The listing builds one solid part. Answer for the finished solid, in the listing's coordinates (mm). Round coordinates to 2 decimals unless told otherwise and drop trailing zeros. Loops run counter-clockwise (first coordinate to the right, second up) from the corner with the lowest first, then second, coordinate; pieces in that order, holes last. Notation, with made-up numbers: (30, -18.75) - (82, -18.75) arc R15 ccw to (82, -8.75) - close; hole circle Ø8 at (75, 89). An arc over 180 degrees is marked (long way). One line per item, written item: value.
```python
from build123d import *

# Parameters (mm, degrees)
SKETCH1_2_R         = 1.6383
SKETCH1_2_R_2       = 0.8382
BOSS_EXTRUDE2_DEPTH = 1.575


with BuildPart() as part:
    # Sketch1_2 → Boss-Extrude2 (new body)
    with BuildSketch(Plane(origin=(0, 0, 0), x_dir=(1, 0, 0), z_dir=(0, 1, 0))):
        with BuildLine():
            Line((-38.39500299, 29.999999735), (-42.73000299, 29.999999735))
            Line((-42.73000299, 29.999999735), (-43.011025994, 30.003097626))
            ThreePointArc((-43.011025994, 30.003097626), (-43.710996344, 30.299838092), (-44.000003042, 31.003036872))
            Line((-44.000003042, 31.003036872), (-44.000003042, 31.269999735))
            Line((-44.000003042, 31.269999735), (-44.000005679, 44.999999735))
            ThreePointArc((-44.000005679, 44.999999735), (-43.414218633, 46.414215608), (-42.000002924, 47.000003051))
            Line((-42.000002924, 47.000003051), (-30.435003, 47.000003051))
            Line((-30.435003, 47.000003051), (-30.435003, 22.255357341))
            Line((-30.435003, 22.255357341), (-11.909003, 22.255357341))
            Line((-11.909003, 22.255357341), (-11.909003, -8.5))
            Line((-11.909003, -8.5), (-23.409003, -8.5))
            Line((-23.409003, -8.5), (-23.409003, -31.499996949))
            Line((-23.409003, -31.499996949), (23.408997, -31.499996949))
            Line((23.408997, -31.499996949), (23.408997, -8.499997555))
            Line((23.408997, -8.499997555), (11.97084713, -8.499997555))
            Line((11.97084713, -8.499997555), (11.97084713, 22.255357341))
            Line((11.97084713, 22.255357341), (30.434997, 22.255357341))
            Line((30.434997, 22.255357341), (30.434997, 47.000003051))
            Line((30.434997, 47.000003051), (42.000008541, 47.000003051))
            ThreePointArc((42.000008541, 47.000003051), (43.414213215, 46.414220704), (43.999996956, 45.000016607))
            Line((43.999996956, 45.000016607), (43.999996956, 32.000003378))
            Line((43.999996956, 32.000003378), (43.999996956, 31.015615364))
            ThreePointArc((43.999996956, 31.015615364), (43.706534093, 30.307939396), (42.998386406, 30.015616661))
            Line((42.998386406, 30.015616661), (33.825607551, 30.030389905))
            ThreePointArc((33.825607551, 30.030389905), (33.117459864, 29.738067169), (32.823997, 29.030391202))
            Line((32.823997, 29.030391202), (32.823997, -30.453996949))
            ThreePointArc((32.823997, -30.453996949), (33.116890219, -31.16110373), (33.823997, -31.453996949))
            Line((33.823997, -31.453996949), (36.099999555, -31.453996949))
            Line((36.099999555, -31.453996949), (42.849728118, -31.453996949))
            ThreePointArc((42.849728118, -31.453996949), (43.556834899, -31.746890168), (43.849728118, -32.453996949))
            Line((43.849728118, -32.453996949), (43.849728118, -36.999996949))
            Line((43.849728118, -36.999996949), (43.849728118, -46.999996949))
            Line((43.849728118, -46.999996949), (-42.000000178, -46.999996949))
            ThreePointArc((-42.000000178, -46.999996949), (-43.414212804, -46.414211581), (-44.000000499, -44.999999921))
            Line((-44.000000499, -44.999999921), (-44.000000178, -38.976999921))
            Line((-44.000000178, -38.976999921), (-44.000000178, -32.453999802))
            ThreePointArc((-44.000000178, -32.453999802), (-43.70710696, -31.746893021), (-43.000000178, -31.453999802))
            Line((-43.000000178, -31.453999802), (-36.100000549, -31.453999802))
            Line((-36.100000549, -31.453999802), (-33.824003042, -31.453999802))
            ThreePointArc((-33.824003042, -31.453999802), (-33.116896261, -31.161106583), (-32.824003042, -30.453999802))
            Line((-32.824003042, -30.453999802), (-32.824003042, 29.011483943))
            ThreePointArc((-32.824003042, 29.011483943), (-33.117785331, 29.719478678), (-33.826516131, 30.011480785))
            Line((-33.826516131, 30.011480785), (-38.39500299, 29.999999735))
        make_face()
        with Locations(Location((40, 43.5, 0), (0, 0, 270))):
            Circle(SKETCH1_2_R, mode=Mode.SUBTRACT)
        with Locations(Location((-40, 43.5, 0), (0, 0, 270))):
            Circle(SKETCH1_2_R, mode=Mode.SUBTRACT)
        with Locations(Location((-37.6, -42.2, 0), (0, 0, 270))):
            Circle(SKETCH1_2_R, mode=Mode.SUBTRACT)
        with Locations(Location((36.1, -42.2, 0), (0, 0, 270))):
            Circle(SKETCH1_2_R, mode=Mode.SUBTRACT)
        with Locations(Location((-36.785003, 36.350003051, 0), (0, 0, 270))):
            Circle(SKETCH1_2_R_2, mode=Mode.SUBTRACT)
        with Locations(Location((-26.220003, 17.93193176, 0), (0, 0, 270))):
            Circle(SKETCH1_2_R_2, mode=Mode.SUBTRACT)
        with Locations(Location((26.219997, 17.93193176, 0), (0, 0, 270))):
            Circle(SKETCH1_2_R_2, mode=Mode.SUBTRACT)
        with Locations(Location((36.784997, 36.368003051, 0), (0, 0, 270))):
            Circle(SKETCH1_2_R_2, mode=Mode.SUBTRACT)
    extrude(amount=BOSS_EXTRUDE2_DEPTH)


solid = part.part
```
1) A cutting plane is placed at D-D on z = -25. Give the vertices of the cut face in (x, y) (3 decimals).
Final values:
outline: (-32.824, 0) - (-30.435, 0) - (-30.435, 1.575) - (-32.824, 1.575) - close; (30.435, 0) - (32.824, 0) - (32.824, 1.575) - (30.435, 1.575) - close
2) A cutting plane is placed at A-A on z = 42.2. Give the vertices of the cut face in (x, y) (3 decimals).
Final values:
outline: (-44, 0) - (-39.238, 0) - (-39.238, 1.575) - (-44, 1.575) - close; (-35.962, 0) - (34.462, 0) - (34.462, 1.575) - (-35.962, 1.575) - close; (37.738, 0) - (43.85, 0) - (43.85, 1.575) - (37.738, 1.575) - close
3) A cutting plane is placed at C-C on x = 40. Give the vertices of the cut face in (y, z) (3 decimals), and give its area (3 significant figures).
Final values:
outline: (0, -47) - (1.575, -47) - (1.575, -45.138) - (0, -45.138) - close; (0, -41.862) - (1.575, -41.862) - (1.575, -30.02) - (0, -30.02) - close; (0, 31.454) - (1.575, 31.454) - (1.575, 47) - (0, 47) - close
area: 46.1 mm2
4) Consider L1, parallel to X at y = 0.75, z = -35 (3 decimals); L2, parallel to Z at x = 19, y = 0.3; L3, parallel to X at y = 0.65, z = -9.5. Determine where each line is inside the solid, lowest interval first.
Final values:
L1: -44 to -30.435, 30.435 to 44
L2: -22.26 to 8.5, 31.5 to 47
L3: -32.82 to -11.91, 11.97 to 32.82
5) For a pull along Z with two mould halves and no side action, classify faces 1 (the cylindrical face through (37.724, 0.776, 41.987)), 2 (the cylindrical face through (-43.43, 0.78, -46.4)), 3 (the flat face through (-13, 0, 7)) as released by +Z, released by -Z, zero draft, split by the parting line, or undercut.
Final values:
face 1: undercut
face 2: released by -Z
face 3: zero draft
6) Each of these flat-tipped pins is pushed along its axis until it touches: pin 1 Ø0.8 at (y, z) = (1, 16.5) entering from +X; pin 2 Ø1.5 at (x, z) = (-26.22, -17.93) entering from +Y; pin 3 Ø1.9 at (x, z) = (36.78, -36.37) entering from -Y; pin 4 Ø0.5 at (x, y) = (-20, 1) entering from -Z. Where does it stop, or does it pass through?
Final values:
pin 1: x = 32.82
pin 2: through
pin 3: y = 0
pin 4: z = -22.26
7) A cutting plane is placed at B-B on z = -43.5. Give the vertices of the cut face in (x, y) (3 decimals), and give its area (3 significant figures).
Final values:
outline: (-44, 0) - (-41.638, 0) - (-41.638, 1.575) - (-44, 1.575) - close; (-38.362, 0) - (-30.435, 0) - (-30.435, 1.575) - (-38.362, 1.575) - close; (30.435, 0) - (38.362, 0) - (38.362, 1.575) - (30.435, 1.575) - close; (41.638, 0) - (44, 0) - (44, 1.575) - (41.638, 1.575) - close
area: 32.4 mm2
